Check sheet for the modelled part. Datum: model origin and axes. Units: mm. Face numbers are marked on the shaded views. A direction names the side the tool comes from. Coordinates: 2 decimals unless noted, no trailing zeros. Write each loop counter-clockwise with the first axis right and the second up, starting at its lowest first coordinate (ties: lowest second). Pieces come first, ordered by that corner, then holes. Notation, with made-up numbers: (39.5, 80.5) - (44.5, 80.5) arc R19 cw to (44.5, 111.5) - close; hole circle Ø9 at (-19, 20.5). An arc over 180 degrees is marked (long way). Use one line per item in the form item = value. Start each with the question number.
1. Cross-section at D-D on x = 27. Record the boundary of the cut face in (y, z), then the cut area to 3 significant figures.
2. Draft check along Y on the marked faces 1, 2, 3 and 4. Enter one of: +Y half, -Y half, draft (parallel to the pull), parting line (faces both ways), or undercut.
3. Scan lines: line 1 along Y through (x, z) = (4.5, 2); line 2 along Y through (x, z) = (-13.5, 7.5); line 3 along X through (y, z) = (72.5, -1). Record each from-to range of solid material in increasing order.
4. Tool access check on the marked faces 5, 6 and 7. Record the directions out of +Z, -Z, +X, -X, +Y, -Y that give a thin tool (end or side, any length) a straight path to the whole face; none if there is none.
5. Cross-section at C-C on y = 24. Record the boundary of the cut face in (x, z).
6. Cross-section at A-A on x = -3.5. Record the boundary of the cut face in (y, z), then the cut area to 3 significant figures.
7. Go/stop test with flat-tipped pins: pin 1 Ø1.5 at (x, y) = (-6.5, 102) entering from -Z; pin 2 Ø10 at (x, z) = (1.5, 10.5) entering from +Y; pin 3 Ø21 at (y, z) = (39, 1) entering from -X; pin 4 Ø6 at (y, z) = (25, 14) entering from +X. Record where each tip stops, or that it passes through.
8. Cross-section at B-B on z = -1.5. Record the boundary of the cut face in (x, y).
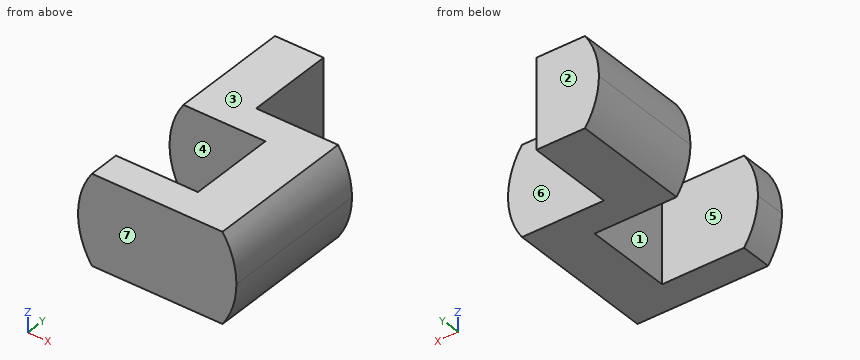
```python
from build123d import *

# Parameters (mm, degrees)
SKETCH1_W           = 76
SKETCH1_H           = 43
BOSS_EXTRUDE1_DEPTH = 15
SKETCH3_W           = 30
SKETCH3_H           = 43
BOSS_EXTRUDE2_DEPTH = 42.1
BOSS_EXTRUDE3_START = 42.1
SKETCH4_W           = 76
SKETCH4_H           = 43
BOSS_EXTRUDE3_DEPTH = 15
SKETCH5_W           = 30
SKETCH5_H           = 43
BOSS_EXTRUDE4_DEPTH = 42.1
CUT_EXTRUDE1_DEPTH  = 114.2


# Read off the part's stored shape, not the designer's step: Cut-Extrude1
with BuildPart() as part:
    # Sketch1 → Boss-Extrude1 (new body)
    with BuildSketch(Plane(origin=(0, 0, 0), x_dir=(1, 0, 0), z_dir=(0, 1, 0))):
        Rectangle(SKETCH1_W, SKETCH1_H)
    extrude(amount=BOSS_EXTRUDE1_DEPTH)

    # Sketch3 → Boss-Extrude2 (add)
    with BuildSketch(Plane(origin=(0, 15, 0), x_dir=(1, 0, 0), z_dir=(0, 1, 0))):
        with Locations((23, 0)):
            Rectangle(SKETCH3_W, SKETCH3_H)
    extrude(amount=BOSS_EXTRUDE2_DEPTH)

    # Sketch4 → Boss-Extrude3 (add)
    with BuildSketch(Plane(origin=(0, 15, 0), x_dir=(1, 0, 0), z_dir=(0, 1, 0)).offset(BOSS_EXTRUDE3_START)):
        Rectangle(SKETCH4_W, SKETCH4_H)
    extrude(amount=BOSS_EXTRUDE3_DEPTH)

    # Sketch5 → Boss-Extrude4 (add)
    with BuildSketch(Plane(origin=(0, 72.1, 0), x_dir=(1, 0, 0), z_dir=(0, 1, 0))):
        with Locations((-23, 0)):
            Rectangle(SKETCH5_W, SKETCH5_H)
    extrude(amount=BOSS_EXTRUDE4_DEPTH)

    # Cut-Extrude1 outline → Cut-Extrude1 (cut)
    with BuildSketch(Plane(origin=(0, 0, 0), x_dir=(1, 0, 0), z_dir=(0, 1, 0))):
        with BuildLine():
            Line((-38, -21.5), (-31.332890068, -21.5))
            ThreePointArc((-31.332890068, -21.5), (-36.294970902, -11.255002765), (-38, 1.36e-07))
            Line((-38, 1.36e-07), (-38, -21.5))
        make_face()
        with BuildLine():
            Line((-38, 21.5), (-38, 1.36e-07))
            ThreePointArc((-38, 1.36e-07), (-36.294970861, 11.255002895), (-31.332890068, 21.5))
            Line((-31.332890068, 21.5), (-38, 21.5))
        make_face()
        with BuildLine():
            ThreePointArc((38, -1.36e-07), (36.294970861, -11.255002895), (31.332890068, -21.5))
            Line((31.332890068, -21.5), (38, -21.5))
            Line((38, -21.5), (38, -1.36e-07))
        make_face()
        with BuildLine():
            ThreePointArc((31.332890068, 21.5), (36.294970902, 11.255002765), (38, -1.36e-07))
            Line((38, -1.36e-07), (38, 21.5))
            Line((38, 21.5), (31.332890068, 21.5))
        make_face()
    extrude(amount=CUT_EXTRUDE1_DEPTH, mode=Mode.SUBTRACT)


solid = part.part
```
Final values:
q1.outline = (0, -21.5) - (72.1, -21.5) - (72.1, 21.5) - (0, 21.5) - close
q1.area = 3,100 mm²
q2.face_1 = undercut
q2.face_2 = +Y half
q2.face_3 = draft
q2.face_4 = undercut
q3.line_1 = 0 to 15, 57.1 to 72.1
q3.line_2 = 0 to 15, 57.1 to 114.2
q3.line_3 = -37.99 to -8
q4.face_5 = +Z, -Z, -X
q4.face_6 = +Z, -Z, +X, +Y
q4.face_7 = +Z, -Z, +X, -X, -Y
q5.outline = (8, -21.5) - (31.33, -21.5) arc R38 ccw to (31.33, 21.5) - (8, 21.5) - close
q6.outline = (0, -21.5) - (15, -21.5) - (15, 21.5) - (0, 21.5) - close; (57.1, -21.5) - (72.1, -21.5) - (72.1, 21.5) - (57.1, 21.5) - close
q6.area = 1,290 mm²
q7.pin_1 = through
q7.pin_2 = 72.1
q7.pin_3 = 8
q7.pin_4 = 36.37
q8.outline = (-37.97, 0) - (37.97, 0) - (37.97, 72.1) - (-8, 72.1) - (-8, 114.2) - (-37.97, 114.2) - (-37.97, 57.1) - (8, 57.1) - (8, 15) - (-37.97, 15) - close
